CAD build for the part. Positions are in the model's coordinates, mm. Face numbers are marked on the shaded views. A direction names the side the tool comes from. Coordinates: 2 decimals unless noted, no trailing zeros. Write each loop counter-clockwise with the first axis right and the second up, starting at its lowest first coordinate (ties: lowest second). Pieces come first, ordered by that corner, then holes.
Autodesk Fusion 360 part; units mm, degrees
sketch "Schizzo1" plane through (0, 0, 0) normal (0, 0, 1) x (1, 0, 0)
  line L0 (4.4965, 58.7959) -> (119.1965, 58.7959) construction
  line L1 (119.1965, 58.7959) -> (119.1965, 5.0959) construction
  line L2 (119.1965, 5.0959) -> (4.4965, 5.0959) construction
  line L3 (4.4965, 5.0959) -> (4.4965, 58.7959) construction
  line L4 (4.4965, 31.9459) -> (119.1965, 31.9459) construction
  line L5 (61.8465, 58.7959) -> (61.8465, 5.0959) construction
  line L6 (119.0965, 5.1959) -> (4.5965, 5.1959)
  line L7 (4.5965, 5.1959) -> (4.5965, 58.6959)
  line L8 (4.5965, 58.6959) -> (119.0965, 58.6959)
  line L9 (119.0965, 58.6959) -> (119.0965, 5.1959)
  line L10 (117.1965, 7.0959) -> (6.4965, 7.0959)
  line L11 (6.4965, 7.0959) -> (6.4965, 56.7959)
  line L12 (6.4965, 56.7959) -> (117.1965, 56.7959)
  line L13 (117.1965, 56.7959) -> (117.1965, 7.0959)
  line L14 (6.4965, 56.7959) -> (34.4965, 56.7959)
  line L15 (34.4965, 56.7959) -> (34.4965, 46.7959)
  line L16 (34.4965, 46.7959) -> (6.4965, 46.7959)
  line L17 (6.4965, 46.7959) -> (6.4965, 56.7959)
  line L18 (92.9965, 56.7959) -> (92.9965, 46.7959)
  line L19 (92.9965, 46.7959) -> (64.9965, 46.7959)
  line L20 (64.9965, 46.7959) -> (64.9965, 56.7959)
  line L21 (64.9965, 56.7959) -> (92.9965, 56.7959)
  line L22 (4.4965, 36.9459) -> (119.0965, 36.9459)
  line L23 (4.4965, 26.9459) -> (119.0965, 26.9459)
  line L24 (51.8465, 58.7959) -> (51.8465, 5.0959)
  line L25 (61.8465, 58.7959) -> (61.8465, 5.0959)
  dimension "d1" = 114.7
  dimension "d2" = 53.7
  dimension "d3" = 0.1
  dimension "d6" = 2
  dimension "d7" = 28
  dimension "d8" = 10
  dimension "d11" = 58.5
  dimension "d12" = 0
  dimension "d15" = 10
  dimension "d23" = 10
extrude "Estrusione1" add sketch "Schizzo1" along normal blind 1 contours L10 L13 L23 L25 | L10 L23 L24 L25 | L13 L22 L23 L25 | L10 L11 L23 L24 | L22 L23 L24 L25 | L12 L13 L18 L19 L20 L22 L25 | L11 L22 L23 L24 | L12 L22 L24 L25 | L11 L12 L15 L16 L22 L24
extrude "Estrusione2" add sketch "Schizzo1" along normal blind 4 contours L6 L9 L10 L13 L23 L25 | L6 L10 L24 L25 | L9 L13 L22 L23 | L6 L7 L10 L11 L23 L24 | L8 L9 L12 L13 L21 L22 L25 | L13 L22 L23 L25 | L22 L23 L24 L25 | L7 L11 L22 L23 | L11 L22 L23 L24 | L8 L12 L24 L25 | L7 L8 L11 L12 L14 L17 L22 L24
fillet "Raccordo1" radius 2 4 edges at (4.5965, 5.1959, 2) (119.0965, 5.1959, 2) (119.0965, 58.6959, 2) (4.5965, 58.6959, 2)
ref_plane "Piano di lavoro1" through (61.8465, 31.9459, 0) normal (-1, 0, 0) x (0, -1, 0)
sketch "Schizzo3" plane through (61.8465, 0, 0) normal (-1, 0, 0) x (0, -1, 0)
  line L0 (-26.9459, 4) -> (-36.9459, 4) construction
  line L1 (-36.9459, 4) -> (-36.9459, 0) construction
  line L2 (-36.9459, 0) -> (-26.9459, 0) construction
  line L3 (-26.9459, 0) -> (-26.9459, 4) construction
  line L4 (-56.6959, 4) -> (-7.1959, 4) construction
  line L5 (-58.7959, 0) -> (-5.0959, 0) construction
  line L6 (-26.9459, 1) -> (-26.9459, 4) construction
  line L7 (-36.9459, 1) -> (-36.9459, 4) construction
  line L8 (-31.9459, 4) -> (-31.9459, 0) construction
  line L9 (-26.9459, 1) -> (-36.9459, 1) construction
  line L10 (-26.9459, 1) -> (-26.9459, 4)
  line L11 (-26.9459, 4) -> (-28.678, 1)
  line L12 (-28.678, 1) -> (-26.9459, 1)
  line L13 (-36.9459, 1) -> (-36.9459, 4)
  line L14 (-36.9459, 4) -> (-35.2139, 1)
  line L15 (-35.2139, 1) -> (-36.9459, 1)
  dimension "d20" = 30
extrude "Estrusione4" cut sketch "Schizzo3" along normal mid plane 110
extrude "Estrusione5" add sketch "Schizzo1" along normal blind 2 contours L6 L10 L24 L25 | L10 L23 L24 L25 | L22 L23 L24 L25 | L12 L22 L24 L25 | L8 L12 L24 L25
sketch "Schizzo4" plane through (0, 0, 4) normal (0, 0, 1) x (-1, 0, 0)
  arc A0 (-6.5965, -58.6959) -> (-4.5965, -56.6959) centre (-6.5965, -56.6959) ccw
  line L0 (-4.5965, -56.6959) -> (-4.5965, -7.1959)
  arc A1 (-4.5965, -7.1959) -> (-6.5965, -5.1959) centre (-6.5965, -7.1959) ccw
  line L1 (-6.5965, -5.1959) -> (-117.0965, -5.1959)
  arc A2 (-117.0965, -5.1959) -> (-119.0965, -7.1959) centre (-117.0965, -7.1959) ccw
  line L2 (-119.0965, -7.1959) -> (-119.0965, -56.6959)
  arc A3 (-119.0965, -56.6959) -> (-117.0965, -58.6959) centre (-117.0965, -56.6959) ccw
  line L3 (-117.0965, -58.6959) -> (-6.5965, -58.6959)
  line L4 (-117.1965, -36.9459) -> (-116.8465, -36.9459)
  line L5 (-116.8465, -36.9459) -> (-6.8465, -36.9459)
  line L6 (-6.8465, -36.9459) -> (-6.4965, -36.9459)
  line L7 (-6.4965, -36.9459) -> (-6.4965, -56.7959)
  line L8 (-6.4965, -56.7959) -> (-117.1965, -56.7959)
  line L9 (-117.1965, -56.7959) -> (-117.1965, -36.9459)
  line L10 (-117.1965, -7.0959) -> (-6.4965, -7.0959)
  line L11 (-6.4965, -7.0959) -> (-6.4965, -26.9459)
  line L12 (-6.4965, -26.9459) -> (-6.8465, -26.9459)
  line L13 (-6.8465, -26.9459) -> (-116.8465, -26.9459)
  line L14 (-116.8465, -26.9459) -> (-117.1965, -26.9459)
  line L15 (-117.1965, -26.9459) -> (-117.1965, -7.0959)
  line L16 (-4.5965, -58.6959) -> (-119.0965, -58.6959) construction
  line L17 (-119.0965, -58.6959) -> (-119.0965, -5.1959) construction
  line L18 (-119.0965, -5.1959) -> (-4.5965, -5.1959) construction
  line L19 (-4.5965, -5.1959) -> (-4.5965, -58.6959) construction
  line L20 (-49.1965, -58.6959) -> (-58.1965, -58.6959)
  line L21 (-58.1965, -58.6959) -> (-58.1965, -5.1959)
  line L22 (-58.1965, -5.1959) -> (-49.1965, -5.1959)
  line L23 (-49.1965, -5.1959) -> (-49.1965, -58.6959)
  line L24 (-65.1965, -58.6959) -> (-74.1965, -58.6959)
  line L25 (-74.1965, -58.6959) -> (-74.1965, -5.1959)
  line L26 (-74.1965, -5.1959) -> (-65.1965, -5.1959)
  line L27 (-65.1965, -5.1959) -> (-65.1965, -58.6959)
  line L28 (-53.6965, -58.6959) -> (-53.6965, -5.1959) construction
  line L29 (-69.6965, -58.6959) -> (-69.6965, -5.1959) construction
  line L30 (-2.6965, -58.6959) -> (-2.6965, -5.1959) construction
  dimension "d28" = 9
  dimension "d29" = 9
  dimension "d33" = 1.9
  dimension "d34" = 51
  dimension "d35" = 67
extrude "Estrusione6" cut sketch "Schizzo4" against normal blind 2 contours L3 L8 L20 L21 L23 | L5 L8 L21 L23 | L3 L8 L24 L25 L27 | L5 L13 L21 L23 | L1 L10 L21 L22 L23 | L5 L8 L25 L27 | L10 L13 L21 L23 | L5 L13 L25 L27 | L1 L10 L25 L26 L27 | L10 L13 L25 L27
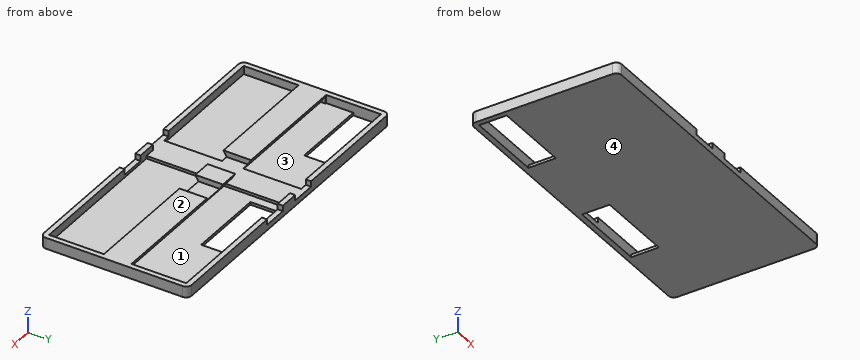
Item 1: Two-plate mould, pull along Y, no slides. Class the marked faces 3 and 4: +Y half, -Y half, draft (parallel to the pull), parting line (faces both ways), or undercut.
Item 2: Which spindle directions (+Z, -Z, +X, -X, +Y, -Y) get a long thin tool onto all of the face, cutting with end or side? Do the marked faces 1 and 2. Say none if no direction does.
Item 3: Saw through at B-B, the plane x = 90.5. Write the cut outline in (y, z).
Item 4: Saw through at C-C, the plane x = 37. Write the cut outline in (y, z), and give its area (3 significant figures).
Item 5: Wall check: line 1 along X through (y, z) = (55.5, 0.6); line 2 along X through (y, z) = (30, 3.5); line 3 along X through (y, z) = (53.5, 2.9). Give the ranges that are in metal, low to high.
Item 6: Saw through at A-A, the plane y = 55.5. Write the cut outline in (x, z), and give its area (3 significant figures).
Item 7: Saw through at D-D, the plane y = 33. Write the cut outline in (x, z).
Item 8: Flat gauge pins, fed straight in: pin 1 Ø1.5 at (y, z) = (58, 3) entering from -X; pin 2 Ø11 at (x, y) = (98, 17) entering from +Z; pin 3 Ø1.5 at (x, y) = (47, 13.5) entering from -Z; pin 4 Ø4 at (x, y) = (70, 31) entering from +Z. Where does each tip first touch, or does it go through?
Working result:
1. face 3: undercut
1. face 4: draft
2. face 1: none
2. face 2: +Z, +X, -X, +Y, -Y
3. outline: (5.2, 0) - (46.8, 0) - (46.8, 1) - (35.21, 1) - (36.95, 4) - (26.95, 4) - (28.68, 1) - (7.1, 1) - (7.1, 4) - (5.2, 4) - close; (56.8, 0) - (58.7, 0) - (58.7, 4) - (56.8, 4) - close
4. outline: (5.2, 0) - (58.7, 0) - (58.7, 4) - (56.8, 4) - (56.8, 1) - (35.21, 1) - (36.95, 4) - (26.95, 4) - (28.68, 1) - (7.1, 1) - (7.1, 4) - (5.2, 4) - close
4. area: 89.7 mm2
5. line 1: x = 4.6 to 6.5, 34.5 to 65, 93 to 119.1
5. line 2: x = 4.6 to 49.2, 58.2 to 65.2, 74.2 to 119.1
5. line 3: x = 4.6 to 6.5, 117.2 to 119.1
6. outline: (4.6, 0) - (6.5, 0) - (6.5, 4) - (4.6, 4) - close; (34.5, 0) - (65, 0) - (65, 1) - (61.85, 1) - (61.85, 2) - (51.85, 2) - (51.85, 1) - (34.5, 1) - close; (93, 0) - (119.1, 0) - (119.1, 4) - (117.2, 4) - (117.2, 1) - (93, 1) - close
6. area: 79.9 mm2
7. outline: (4.6, 0) - (119.1, 0) - (119.1, 4) - (74.2, 4) - (74.2, 2) - (65.2, 2) - (65.2, 4) - (58.2, 4) - (58.2, 2) - (49.2, 2) - (49.2, 4) - (4.6, 4) - close
8. pin 1: stops at x = 4.67
8. pin 2: stops at z = 1
8. pin 3: stops at z = 0
8. pin 4: stops at z = 2
